```python
from build123d import *

# Parameters (mm, degrees)
SKETCH1_R           = 10
SKETCH1_R_2         = 1.5
SKETCH1_R_3         = 20
BOSS_EXTRUDE1_DEPTH = 3


with BuildPart() as part:
    # Sketch1 → Boss-Extrude1 (new body)
    with BuildSketch(Plane.XY):
        with BuildLine():
            ThreePointArc((45, 0), (0, 45), (-45, 0))
            Line((-45, 0), (-43.785466077, -10.384265038))
            Line((-43.785466077, -10.384265038), (-25, -171))
            ThreePointArc((-25, -171), (0, -196), (25, -171))
            Line((25, -171), (43.785466077, -10.384265038))
            Line((43.785466077, -10.384265038), (45, 0))
        make_face()
        with Locations((0, -171)):
            Circle(SKETCH1_R, mode=Mode.SUBTRACT)
        with Locations((-34.641016151, -20)):
            Circle(SKETCH1_R_2, mode=Mode.SUBTRACT)
        with Locations((0, -40)):
            Circle(SKETCH1_R_2, mode=Mode.SUBTRACT)
        with Locations((-34.641016151, 20)):
            Circle(SKETCH1_R_2, mode=Mode.SUBTRACT)
        Circle(SKETCH1_R_3, mode=Mode.SUBTRACT)
        with Locations((0, 40)):
            Circle(SKETCH1_R_2, mode=Mode.SUBTRACT)
        with Locations((34.641016151, -20)):
            Circle(SKETCH1_R_2, mode=Mode.SUBTRACT)
        with Locations((34.641016151, 20)):
            Circle(SKETCH1_R_2, mode=Mode.SUBTRACT)
    extrude(amount=BOSS_EXTRUDE1_DEPTH)


solid = part.part
```
CAD build for the part. Positions are in the model's coordinates, mm. Coordinates: 2 decimals unless noted, no trailing zeros. Order: outer loops, then holes, each group sorted by start corner. A loop starts at its lowest first (then second) coordinate and runs counter-clockwise, first axis right, second up. Notation, with made-up numbers: (60.5, -30) -> (117.5, -30) arc R21 ccw to (117.5, -3) -> close; hole circle Ø1 at (77.5, -6.5). An arc over 180 degrees is marked (long way). Use one line per item in the form item = value. Start each with the question number.
1) Pull direction Z, two halves, no side cores. Call faces 1 (the flat face through (-1, -74, 0)), 2 (the flat face through (-1, -74, 3)), 3 (the cylindrical face through (-0.55, -195.994, 1.479)): +Z half, -Z half, draft (parallel to the pull), parting line (faces both ways), or undercut.
2) Band-saw the part on C-C on y = -25.5. Give the cut face in (x, z), then the cut area to 3 significant figures.
3) Drop a flat-ended pin along its axis: pin 1 (1 mm diameter, centred on x = -13, z = 1.5, fed in from +Y). Give the stop position or say it passes through.
4) Band-saw the part on A-A on z = 2.1. State how many separate pieces and enclosed holes the cut face has, then the cut area to 3 significant figures.
5) Band-saw the part on B-B on x = -5. Give the cut face in (y, z).
6) Band-saw the part on D-D on y = -93. Give the cut face in (x, z), then the cut area to 3 significant figures.
7) Drill centre lines: L1, parallel to Y at x = 0, z = 1.7; L2, parallel to X at y = -21, z = 1.05; L3, parallel to Y at x = -9, z = 2.25. Where is each one in solid material? Low to high. Write a range as [from, to].
Entries:
q1.face_1 = -Z half
q1.face_2 = +Z half
q1.face_3 = draft
q2.outline = (-42.02, 0) -> (42.02, 0) -> (42.02, 3) -> (-42.02, 3) -> close
q2.area = 252 mm2
q3.pin_1 = 43.23
q4.separate_pieces = 1
q4.enclosed_holes = 8
q4.area = 14,500 mm2
q5.outline = (-195.49, 0) -> (-179.66, 0) -> (-179.66, 3) -> (-195.49, 3) -> close; (-162.34, 0) -> (-19.36, 0) -> (-19.36, 3) -> (-162.34, 3) -> close; (19.36, 0) -> (44.72, 0) -> (44.72, 3) -> (19.36, 3) -> close
q6.outline = (-34.12, 0) -> (34.12, 0) -> (34.12, 3) -> (-34.12, 3) -> close
q6.area = 205 mm2
q7.L1 = [-196, -181], [-161, -41.5], [-38.5, -20], [20, 38.5], [41.5, 45]
q7.L2 = [-42.54, -35.76], [-33.52, 33.52], [35.76, 42.54]
q7.L3 = [-194.32, -175.36], [-166.64, -17.86], [17.86, 44.09]
